Autodesk Inventor part; units mm, degrees
ref_plane "YZ Plane" through (0, 0, 0) normal (1, 0, 0) x (0, 1, 0)
ref_plane "XZ Plane" through (0, 0, 0) normal (0, 1, 0) x (-1, 0, 0)
ref_plane "XY Plane" through (0, 0, 0) normal (0, 0, 1) x (1, 0, 0)
sketch "Sketch1" plane through (0, 0, 0) normal (1, 0, 0) x (0, 1, 0)
  circle A0 centre (0, 0) radius 20
  line L0 (8.5, 8.5) -> (-16.9, 8.5)
  line L1 (8.5, 8.5) -> (8.5, -16.9)
  line L2 (0, 0) -> (0, 20)
  line L3 (0, 20) -> (-60.9241, 20)
  line L4 (-60.9241, 20) -> (-60.9241, 18.5)
  line L5 (-60.9241, 18.5) -> (0, 18.5)
  line L6 (0, 18.5) -> (0, 20)
  line L7 (0, 0) -> (14.1421, 14.1421)
  line L8 (0, 0) -> (20, 0)
  line L9 (-16.9, 8.5) -> (-16.9, 18.5)
  line L10 (-16.9, 8.5) -> (-22.9, 14.5)
  line L11 (-22.9, 14.5) -> (-22.9, 18.5)
  line L12 (12.3744, 12.3744) -> (12.1502, 13.2109)
  line L13 (11.3137, 13.435) -> (9.2071, 11.3284)
  line L14 (9.4313, 10.4919) -> (10.2678, 10.2678)
  line L15 (8.5, 8.5) -> (8.5, -16.9)
  line L16 (20, 0) -> (20, -60.9241)
  line L17 (20, -60.9241) -> (18.5, -60.9241)
  line L18 (18.5, -60.9241) -> (18.5, 0)
  line L19 (8.5, -16.9) -> (18.5, -16.9)
  line L20 (8.5, -16.9) -> (14.5, -22.9)
  line L21 (14.5, -22.9) -> (18.5, -22.9)
  arc A1 (9.2071, 11.3284) -> (9.4313, 10.4919) centre (9.5607, 10.9749) ccw
  arc A2 (12.1502, 13.2109) -> (11.3137, 13.435) centre (11.6673, 13.0815) ccw
  line L22 (10.4311, 10.4311) -> (9.483, 10.6851)
  arc A3 (9.3485, 11.187) -> (9.483, 10.6851) centre (9.5607, 10.9749) ccw
  line L23 (9.3485, 11.187) -> (11.4551, 13.2936)
  arc A4 (11.957, 13.1591) -> (11.4551, 13.2936) centre (11.6673, 13.0815) ccw
  line L24 (11.957, 13.1591) -> (12.2111, 12.2111)
  point P0 (0, 8.5)
  point P1 (-17.7041, 9.3041)
  point P2 (-16.9, 10.6953)
  dimension "d0" = 40
  dimension "d1" = 25.4
  dimension "d2" = 1.5
  dimension "d4" = 45
  dimension "d6" = 45
  dimension "d7" = 4
  dimension "d8" = 10
  dimension "d10" = 2.5
  dimension "d11" = 2.5
  dimension "d12" = 60
  dimension "d13" = 1.5
  dimension "d15" = 0.5
  dimension "d16" = 0.2
extrude "Extrusion1" add sketch "Sketch1" along normal blind 264 contours L7 L12 A2 L13 A1 L14 L0 L2 A0 | L7 L24 A4 L23 A3 L22 L14 A1 L13 A2 L12 | L5 L2 L0 L9 A0 | A0 L9 L5 | L7 L22 A3 L23 A4 L24 | L9 L10 A0 | A0 L10 L11 L5 L9
sketch "Sketch2" plane through (0, -22.9, 18.5) normal (0, 0, 1) x (1, 0, 0)
  line L0 (0, 22.9) -> (0, 0)
  line L1 (0, 0) -> (264, 0)
  line L2 (264, 22.9) -> (264, 0)
  line L3 (0, 22.9) -> (264, 22.9)
  line L4 (38.3257, 13.1) -> (36.6514, 16)
  line L5 (36.6514, 16) -> (38.3257, 18.9)
  line L6 (38.3257, 18.9) -> (41.6743, 18.9)
  line L7 (41.6743, 18.9) -> (43.3486, 16)
  line L8 (43.3486, 16) -> (41.6743, 13.1)
  line L9 (41.6743, 13.1) -> (38.3257, 13.1)
  line L10 (0, 6) -> (264, 6)
  circle A0 centre (40, 16) radius 1.65
  dimension "d20" = 10
  dimension "d21" = 5.8
  dimension "d22" = 40
  dimension "d25" = 3.3
extrude "Extrusion2" cut sketch "Sketch2" against normal blind 6 contours L4 L5 L6 L7 L8 L9 | A0
extrude "Extrusion3" cut sketch "Sketch2" against normal through all contours A0
sketch "Sketch3" plane through (0, -22.9, 18.5) normal (0, 0, 1) x (1, 0, 0)
  line L0 (0, 37.0421) -> (264, 37.0421)
  line L1 (0, 0) -> (264, 0)
  line L2 (0, 22.9) -> (0, 0)
  line L3 (0, 22.9) -> (0, 37.0421)
  line L4 (2.4384, 37.0421) -> (17.8575, 0)
  line L5 (0, 0) -> (264, 0)
  line L6 (2.4384, 37.0421) -> (0, 42.9)
  point P0 (0, 26.9698)
  dimension "d28" = 112.6
sketch "Sketch4" plane through (264, 14.1421, 14.1421) normal (0, 0.7071, -0.7071) x (-1, 0, 0)
  line L0 (264, 0) -> (0, 0)
  line L1 (0, -7.9792) -> (0, 0)
  line L2 (264, -7.9792) -> (0, -7.9792)
  circle A0 centre (234, -4) radius 1.5
  line L3 (264, -7.9792) -> (264, 0)
  line L4 (132, -7.9792) -> (132, 0)
  ellipse E0 centre (224, -18.8686) end of major axis (222.35, -18.8686) minor radius 1.1667
  point P0 (264, -20)
  dimension "d34" = 3
  dimension "d35" = 4
  dimension "d46" = 30
extrude "Extrusion5" cut sketch "Sketch4" against normal blind 3 contours A0
ref_plane "Work Plane1" through (132, 0, 0) normal (-1, 0, 0) x (0, 0, 1)
mirror "Mirror1" about plane through (132, 0, 0) normal (-1, 0, 0) of "Extrusion5", "Extrusion2", "Extrusion3"
properties part number "ESQUINA_REDONDEADA_R20" material "Steel, Mild, Welded"
Here's how the part is built. I have some questions about the finished solid (model axes, mm). A direction names the side the tool comes from. Coordinates: 2 decimals unless noted, no trailing zeros. Write each loop counter-clockwise with the first axis right and the second up, starting at its lowest first coordinate (ties: lowest second). Pieces come first, ordered by that corner, then holes. Notation, with made-up numbers: (63.25, -15) -> (107.25, -15) arc R28 cw to (107.25, 8) -> close; hole circle Ø11 at (16.25, 56). An arc over 180 degrees is marked (long way). Use a Markdown table: item, result. Add a question column.
(1) For faces 1 (the flat face through (225.4, -5.6, 12.5)), 2 (the cylindrical face through (130.2, 7.6, 18.5)), which set-ups out of +Z, -Z, +X, -X, +Y, -Y let a thin tool reach every point of the face, with its end or its side?
(2) I'm going to push flat-ended pins straight in: P1, Ø1.7, axis at x = 223.5, y = -8.5, coming from the +Z side; P2, Ø1, axis at x = 204.5, y = 0.5, coming from the +Z side; P3, Ø1, axis at x = 187, y = -17, coming from the +Z side; P4, Ø1.6, axis at x = 153, z = 19.5, coming from the -Y side. Where does each tip first touch, or does it pass through?
(3) Please list where these lines run through material, in increasing order: line 1 (Z direction, x = 191, y = -9); line 2 (X direction, y = -6, z = 13.75); line 3 (X direction, y = -8.5, z = 14.75).
(4) If we section it at A-A, the plane x = 47.5: Write out the boundary of the cut face in (y, z), and give its area (3 significant figures).
(5) We'd pull the mould along Z, two halves only. Please class faces 3 (the cylindrical face through (28.57, 10.59, 12.68)), 4 (the flat face through (41.4, -5.6, 12.5)): +Z half, -Z half, draft (parallel to the pull), parting line (faces both ways), or undercut.
Outcome:
| question | item | result |
|---|---|---|
| 1 | face 1 | +Z |
| 1 | face 2 | +Z, +X, -X, +Y |
| 2 | P1 | stops at z = 12.5 |
| 2 | P2 | stops at z = 20 |
| 2 | P3 | stops at z = 18.5 |
| 2 | P4 | stops at y = 0 |
| 3 | line 1 | z = 8.5 to 18.5 |
| 3 | line 2 | x = 0 to 37.17, 42.83 to 221.17, 226.83 to 264 |
| 3 | line 3 | x = 0 to 37.58, 42.42 to 221.58, 226.42 to 264 |
| 4 | outline | (-22.9, 14.5) -> (-16.9, 8.5) -> (8.5, 8.5) -> (14.14, 14.14) arc R20 ccw to (0, 20) -> (0, 18.5) -> (-22.9, 18.5) -> close |
| 4 | area | 332 mm^2 |
| 5 | face 3 | undercut |
| 5 | face 4 | +Z half |
